The listing builds one solid part. Answer for the finished solid, in the listing's coordinates (mm). A direction names the side the tool comes from. Round coordinates to 2 decimals unless told otherwise and drop trailing zeros. Order: outer loops, then holes, each group sorted by start corner. A loop starts at its lowest first (then second) coordinate and runs counter-clockwise, first axis right, second up. Notation, with made-up numbers: (62, 9.25) -> (82, 9.25) arc R22 cw to (82, 47.25) -> close; hole circle Ø11 at (18.5, 32.5). An arc over 180 degrees is marked (long way). Answer in a Markdown table with one row per item. Add a question column.
```python
from build123d import *

# Parameters (mm, degrees)
F0_W      = 1219.2
F0_H      = 609.6
F1_DEPTH  = 1.51892
F2_W      = 1219.2
F2_H      = 609.6
F2_W_2    = 1216.16216
F2_H_2    = 606.56216
F3_DEPTH  = 38.1
F5_DEPTH  = 584.2
F7_W      = 1219.2
F7_H      = 609.6
F8_DEPTH  = 1.51892
F9_W      = 1219.2
F9_H      = 609.6
F9_W_2    = 1213.12432
F9_H_2    = 603.52432
F10_DEPTH = 38.1
F11_W     = 101.6
F11_H     = 609.6
F12_DEPTH = 1.51892
F13_R     = 1.5875
F14_DEPTH = 1.651


# Not quite as in the source:
# - a pattern or mirror of a feature is missing from the dataset's text; its kind, count and spacing are read off the source's solid


with BuildPart() as f1:
    # F0 (on Top) → F1 (new body)
    with BuildSketch(Plane.XY):
        Rectangle(F0_W, F0_H)
    extrude(amount=-F1_DEPTH)

    # F2 (on face) → F3 (join)
    with BuildSketch(Plane(origin=(0, 0, -1.51892), x_dir=(1, 0, 0), z_dir=(0, 0, -1))):
        Rectangle(F2_W, F2_H)
        Rectangle(F2_W_2, F2_H_2, mode=Mode.SUBTRACT)
    extrude(amount=F3_DEPTH)

    # F4 (on face) → F5 (join)
    with BuildSketch(Plane(origin=(0, 0, -1.51892), x_dir=(1, 0, 0), z_dir=(0, 0, -1))):
        Polygon((-571.5, 301.76216), (-571.5, 304.8), (-609.6, 304.8), (-609.6, 266.7), (-606.56216, 266.7), (-606.56216, 301.76216), align=None)
        Polygon((571.5, 304.8), (571.5, 301.76216), (606.56216, 301.76216), (606.56216, 266.7), (609.6, 266.7), (609.6, 304.8), align=None)
    f5 = extrude(amount=F5_DEPTH)

    # F5_copies: F5 across plane
    add(f5.mirror(Plane.ZX))

    # F7 (on offset) → F8 (join)
    with BuildSketch(Plane.XY.offset(-546.1)):
        Rectangle(F7_W, F7_H)
    extrude(amount=-F8_DEPTH)

    # F9 (on face) → F10 (join)
    with BuildSketch(Plane(origin=(0, 0, -547.61892), x_dir=(1, 0, 0), z_dir=(0, 0, -1))):
        Rectangle(F9_W, F9_H)
        Rectangle(F9_W_2, F9_H_2, mode=Mode.SUBTRACT)
    extrude(amount=F10_DEPTH)

    # F11 (on face) → F12 (join)
    with BuildSketch(Plane(origin=(0, 0, -585.71892), x_dir=(1, 0, 0), z_dir=(0, 0, -1))):
        with Locations((-558.8, 0)):
            Rectangle(F11_W, F11_H)
    f12 = extrude(amount=F12_DEPTH)

    # F12_copies: F12 across plane
    add(f12.mirror(Plane(origin=(0, 0, 0), x_dir=(0, 0, 1), z_dir=(1, 0, 0))))

    # F13 (on face) → F14 (cut)
    with BuildSketch(Plane(origin=(0, 0, -587.23784), x_dir=(1, 0, 0), z_dir=(0, 0, -1))):
        with Locations((-584.2, 285.75)):
            Circle(F13_R)
    f14 = extrude(amount=-F14_DEPTH, mode=Mode.SUBTRACT)

    # F14_copies: F14 across plane
    add(f14.mirror(Plane(origin=(0, 0, 0), x_dir=(0, 0, 1), z_dir=(1, 0, 0))), mode=Mode.SUBTRACT)

    # F14_copies1: F14 across plane
    add(f14.mirror(Plane.ZX), mode=Mode.SUBTRACT)

    # F14_copies2: F14 across plane
    add(f14.mirror(Plane(origin=(0, 0, 0), x_dir=(-0.4393852473, 0.8982987278, 0), z_dir=(0.8982987278, 0.4393852473, 0))), mode=Mode.SUBTRACT)


solid = f1.part
```
1. Each of these flat-tipped pins is pushed along its axis until it touches: pin 1 (1.7 mm diameter, centred on x = 275.5, y = 303.5, fed in from -Z); pin 2 (1 mm diameter, centred on x = -324, y = -173.5, fed in from -Z). Where does it stop, or does it pass through?
2. The part is cut by section C-C (x = 336). Give the vertices of the cut face in (y, z).
3. The part is cut by section A-A (y = 0.5). Give the vertices of the cut face in (x, z).
4. The mould has two halves that part along Y. Classify faces 3 (the flat face through (-9, 4, 0)), 4 (the flat face through (606.562, 284, -270)), 5 (the flat face through (-589, -301.762, -270)): released by +Y, released by -Y, zero draft, split by the parting line, or undercut.
5. The part is cut by section B-B (z = -75.5). Give the vertices of the cut face in (x, y).
6. For faces 1 (the flat face through (560, -4, -587.238)), 2 (the flat face through (-589, 301.762, -270)), determine the directions among +Z, -Z, +X, -X, +Y, -Y from which every point of the face is accessible in a straight line to the end or side of a thin tool.
7. Straight lines are drawn through the part: line 1 along Y through (x, z) = (584.2, -586.8); line 2 along Z through (x, y) = (-534.5, 74); line 3 along X through (y, z) = (-285.75, -586.55). For each, find the intervals that lie inside material, in ascending order.
Report:
| question | item | result |
|---|---|---|
| 1 | pin 1 | stops at z = -585.72 |
| 1 | pin 2 | stops at z = -547.62 |
| 2 | outline | (-304.8, -585.72) -> (-301.76, -585.72) -> (-301.76, -547.62) -> (301.76, -547.62) -> (301.76, -585.72) -> (304.8, -585.72) -> (304.8, -546.1) -> (-304.8, -546.1) -> close; (-304.8, -39.62) -> (-303.28, -39.62) -> (-303.28, -1.52) -> (303.28, -1.52) -> (303.28, -39.62) -> (304.8, -39.62) -> (304.8, 0) -> (-304.8, 0) -> close |
| 3 | outline | (-609.6, -587.24) -> (-508, -587.24) -> (-508, -585.72) -> (-606.56, -585.72) -> (-606.56, -547.62) -> (606.56, -547.62) -> (606.56, -585.72) -> (508, -585.72) -> (508, -587.24) -> (609.6, -587.24) -> (609.6, -546.1) -> (-609.6, -546.1) -> close; (-609.6, -39.62) -> (-608.08, -39.62) -> (-608.08, -1.52) -> (608.08, -1.52) -> (608.08, -39.62) -> (609.6, -39.62) -> (609.6, 0) -> (-609.6, 0) -> close |
| 4 | face 3 | zero draft |
| 4 | face 4 | undercut |
| 4 | face 5 | undercut |
| 5 | outline | (-609.6, -304.8) -> (-571.5, -304.8) -> (-571.5, -301.76) -> (-606.56, -301.76) -> (-606.56, -266.7) -> (-609.6, -266.7) -> close; (-609.6, 266.7) -> (-606.56, 266.7) -> (-606.56, 301.76) -> (-571.5, 301.76) -> (-571.5, 304.8) -> (-609.6, 304.8) -> close; (571.5, -304.8) -> (609.6, -304.8) -> (609.6, -266.7) -> (606.56, -266.7) -> (606.56, -301.76) -> (571.5, -301.76) -> close; (571.5, 301.76) -> (606.56, 301.76) -> (606.56, 266.7) -> (609.6, 266.7) -> (609.6, 304.8) -> (571.5, 304.8) -> close |
| 6 | face 1 | -Z, +X, -X, +Y, -Y |
| 6 | face 2 | none |
| 7 | line 1 | y = -304.8 to -287.34, -284.16 to 284.16, 287.34 to 304.8 |
| 7 | line 2 | z = -587.24 to -585.72, -547.62 to -546.1, -1.52 to 0 |
| 7 | line 3 | x = -609.6 to -585.79, -582.61 to -508, 508 to 582.61, 585.79 to 609.6 |
